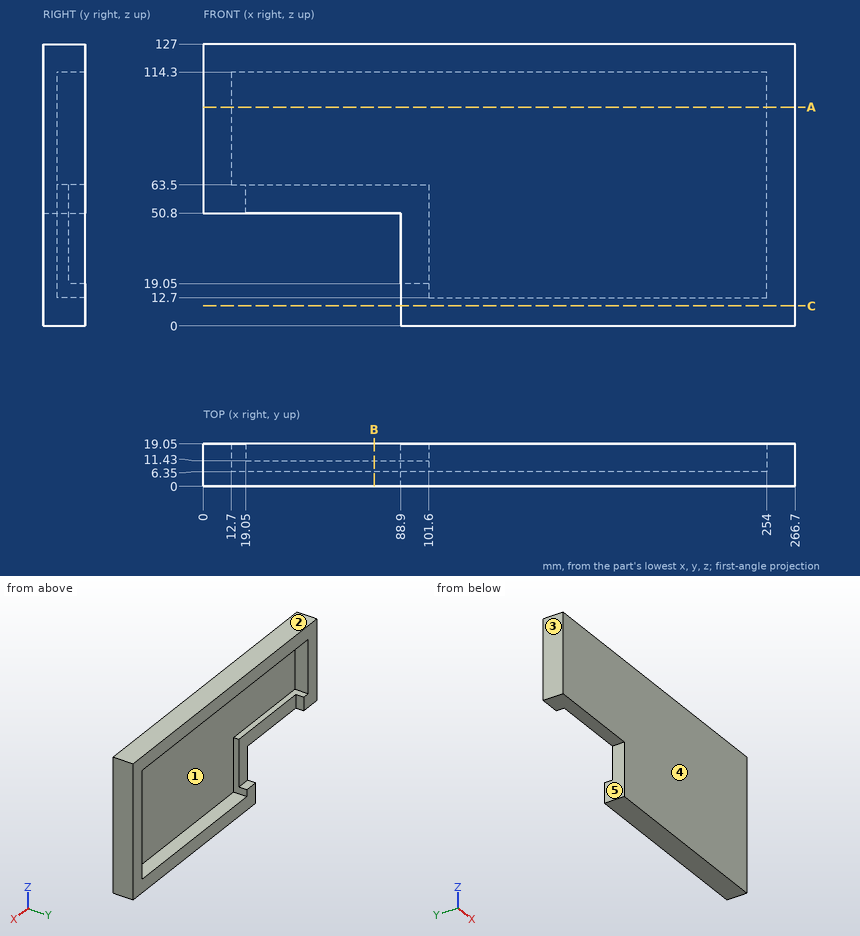
Here's the drawing with two shaded views (mm, measured from the low corner). I have some questions. A direction names the side the tool comes from. Give positions to 0.01 mm unless a question says otherwise; leave off trailing zeros. Write each loop counter-clockwise with the first axis right and the second up, starting at its lowest first coordinate (ties: lowest second). Pieces come first, ordered by that corner, then holes. Notation, with made-up numbers: (-27.5, -17.5) -> (6.5, -17.5) arc R14 cw to (6.5, 6.5) -> close; hole circle Ø8 at (82.5, 51.5). An arc over 180 degrees is marked (long way). Use one line per item in the form item = value. Start each with the question number.
1. On a 3-axis mill with a long thin cutter (end or side, diameter ignored), from which of +Z, -Z, +X, -X, +Y, -Y can I reach the whole of each face in a straight line? I mean the marked faces 4 and 5. Say none if no direction works.
2. Will these pins go through, and if not, where does the flat tip stop? pin 1 Ø5.5 at (y, z) = (10, 37) entering from -X; pin 2 Ø9.5 at (x, y) = (24, 13) entering from -Z.
3. Thinking about a two-plate mould opening in Z: for the marked faces 1, 2 and 3, which applies, +Z half, -Z half, draft (parallel to the pull), parting line (faces both ways), or undercut?
4. Imagine slicing it at A-A on z = 98.5. List the corners of the cut face in (x, y) for me.
5. Imagine slicing it at B-B on x = 77. List the corners of the cut face in (y, z) for me, plus the area to 3 significant figures.
6. If I drill on L1, parallel to Z at x = 99.5, y = 12.25; L2, parallel to Z at x = 160, y = 13; L3, parallel to X at y = 10.25, z = 32, over which ranges is the centre line in solid material (lowest first)?
7. Imagine slicing it at C-C on z = 9. List the corners of the cut face in (x, y) for me, plus the area to 3 significant figures.
Entries:
q1.face_4 = +Z, -Z, +X, -X, -Y
q1.face_5 = -Z, -X, +Y, -Y
q2.pin_1 = 88.9
q2.pin_2 = 50.8
q3.face_1 = undercut
q3.face_2 = +Z half
q3.face_3 = draft
q4.outline = (0, 0) -> (266.7, 0) -> (266.7, 19.05) -> (254, 19.05) -> (254, 6.35) -> (12.7, 6.35) -> (12.7, 19.05) -> (0, 19.05) -> close
q5.outline = (0, 50.8) -> (11.43, 50.8) -> (11.43, 63.5) -> (6.35, 63.5) -> (6.35, 114.3) -> (19.05, 114.3) -> (19.05, 127) -> (0, 127) -> close
q5.area = 710 mm²
q6.L1 = 0 to 19.05, 114.3 to 127
q6.L2 = 0 to 12.7, 114.3 to 127
q6.L3 = 88.9 to 101.6, 254 to 266.7
q7.outline = (88.9, 0) -> (266.7, 0) -> (266.7, 19.05) -> (88.9, 19.05) -> close
q7.area = 3,390 mm²
